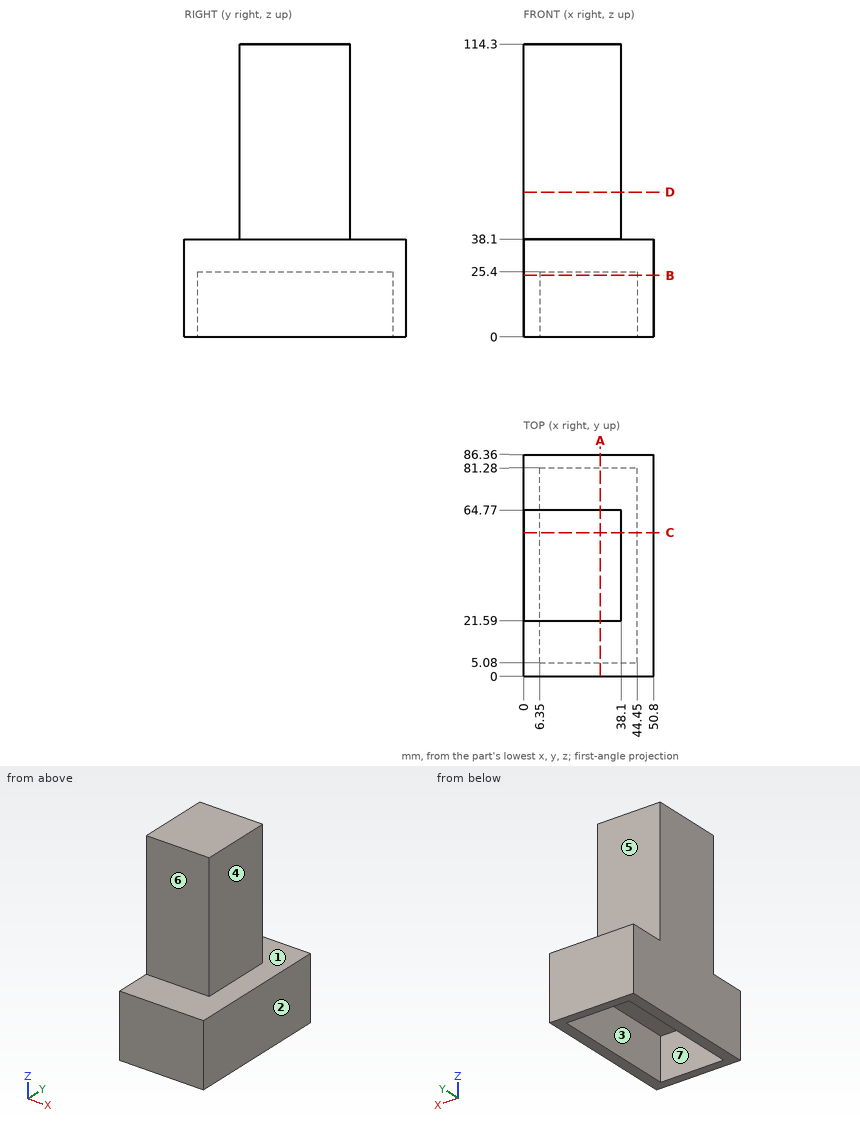
Job drawing, mm, ordinate dimensions from the low corner. One solid piece. A direction names the side the tool comes from. Coordinates: 2 decimals unless noted, no trailing zeros. Order: outer loops, then holes, each group sorted by start corner. A loop starts at its lowest first (then second) coordinate and runs counter-clockwise, first axis right, second up. Notation, with made-up numbers: (77.5, 60) - (82.5, 60) arc R14 ccw to (82.5, 64) - close; hole circle Ø3 at (58.25, 7). An arc over 180 degrees is marked (long way). Write each question's results on one line, items separated by ' | '. Start each with the question number.
Item 1: Flat gauge pins, fed straight in: pin 1 (12 mm diameter, centred on x = 35.5, y = 60, fed in from -Z); pin 2 (19 mm diameter, centred on x = 14, z = 80, fed in from +Y). Where does each tip first touch, or does it go through?
Item 2: Wall check: probe 1 along X at (y, z) = (38.5, 24); probe 2 along Y at (x, z) = (31.5, 8); probe 3 along Z at (x, y) = (3.5, 10). Give the ranges that are in metal, low to high. Write a range as [from, to].
Item 3: Band-saw the part on D-D on z = 56.5. Write the cut outline in (x, y), and give its area (3 significant figures).
Item 4: Band-saw the part on B-B on z = 24. Write the cut outline in (x, y).
Item 5: Band-saw the part on C-C on y = 56. Write the cut outline in (x, z), and give its area (3 significant figures).
Item 6: Band-saw the part on A-A on x = 30. Write the cut outline in (y, z).
Item 7: Tool access for the marked faces 4, 5, 6 and 7: list every direction of +Z, -Z, +X, -X, +Y, -Y with a clear straight run to the whole face (end or side of a thin tool).
Item 8: Mould opens along X. For the marked faces 1, 2 and 3 say: released by +X, released by -X, zero draft, split by the parting line, or undercut.
Numbers:
1) pin 1: z = 25.4 | pin 2: y = 64.77
2) probe 1: [0, 6.35], [44.45, 50.8] | probe 2: [0, 5.08], [81.28, 86.36] | probe 3: [0, 38.1]
3) outline: (0, 21.59) - (38.1, 21.59) - (38.1, 64.77) - (0, 64.77) - close | area: 1,650 mm^2
4) outline: (0, 0) - (50.8, 0) - (50.8, 86.36) - (0, 86.36) - close; hole (6.35, 5.08) - (44.45, 5.08) - (44.45, 81.28) - (6.35, 81.28) - close
5) outline: (0, 0) - (6.35, 0) - (6.35, 25.4) - (44.45, 25.4) - (44.45, 0) - (50.8, 0) - (50.8, 38.1) - (38.1, 38.1) - (38.1, 114.3) - (0, 114.3) - close | area: 3,870 mm^2
6) outline: (0, 0) - (5.08, 0) - (5.08, 25.4) - (81.28, 25.4) - (81.28, 0) - (86.36, 0) - (86.36, 38.1) - (64.77, 38.1) - (64.77, 114.3) - (21.59, 114.3) - (21.59, 38.1) - (0, 38.1) - close
7) face 4: +Z, +X, +Y, -Y | face 5: +Z, +X, -X, +Y | face 6: +Z, +X, -X, -Y | face 7: -Z
8) face 1: zero draft | face 2: released by +X | face 3: undercut
